Can you work these out from the drawing? Everything is in mm from the part's minimum corner. Give positions to 0.01 mm unless a question says otherwise; leave off trailing zeros. Write each loop counter-clockwise with the first axis right and the second up, starting at its lowest first coordinate (ties: lowest second). Pieces come first, ordered by that corner, then holes. Notation, with made-up numbers: (88, 83.5) - (117, 83.5) arc R18 cw to (117, 90.5) - close; hole circle Ø10 at (53, 82). An arc over 180 degrees is marked (long way). Return JSON: item names as keys, results as strings. Group by question number.
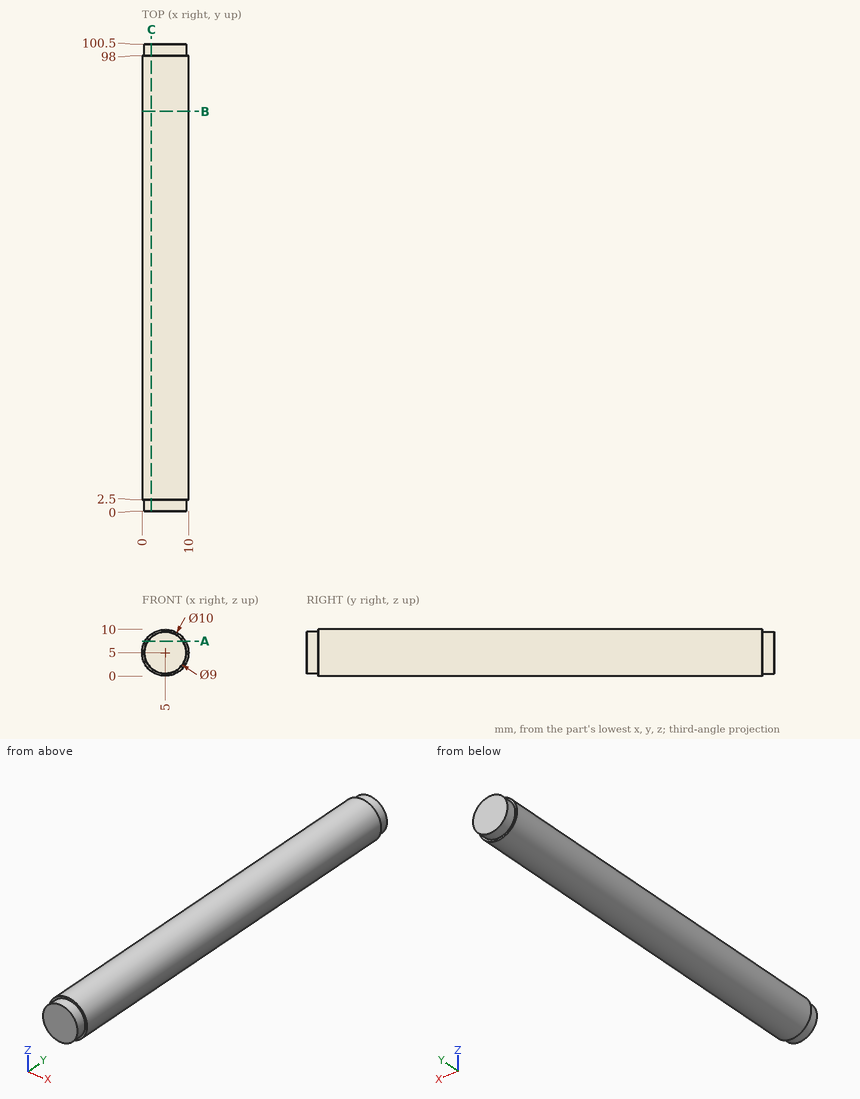
1) I need wall thicknesses on line 1 along Y through (x, z) = (7.5, 9); line 2 along X through (y, z) = (17, 5.25). Which ranges of each line are inside material? Lowest first, please.
2) Imagine slicing it at A-A, the plane z = 7.5. Write out the boundary of the cut face in (x, y), and give its area (3 significant figures).
3) Will these pins go through, and if not, where does the flat tip stop? pin 1 Ø2 at (x, y) = (7, 43) entering from -Z; pin 2 Ø3 at (x, y) = (7, 87.5) entering from +Z; pin 3 Ø3 at (x, y) = (7.5, 36) entering from +Z.
4) Imagine slicing it at B-B, the plane y = 86. Write out the boundary of the cut face in (x, z).
5) Imagine slicing it at C-C, the plane x = 2. Write out the boundary of the cut face in (y, z).
Resolved:
{
 "1": {"line 1": "2.5 to 98", "line 2": "0.01 to 9.99"},
 "2": {"outline": "(0.67, 2.5) - (1.26, 2.5) - (1.26, 0) - (8.74, 0) - (8.74, 2.5) - (9.33, 2.5) - (9.33, 98) - (8.74, 98) - (8.74, 100.5) - (1.26, 100.5) - (1.26, 98) - (0.67, 98) - close", "area": "864 mm^2"},
 "3": {"pin 1": "z = 0.1", "pin 2": "z = 9.97", "pin 3": "z = 9.9"},
 "4": {"outline": "circle Ø10 at (5, 5)"},
 "5": {"outline": "(0, 1.65) - (2.5, 1.65) - (2.5, 1) - (98, 1) - (98, 1.65) - (100.5, 1.65) - (100.5, 8.35) - (98, 8.35) - (98, 9) - (2.5, 9) - (2.5, 8.35) - (0, 8.35) - close"}
}
